Can you work these out from the model? Positions are in its coordinate system, mm. Coordinates: 2 decimals unless noted, no trailing zeros. Order: outer loops, then holes, each group sorted by start corner. A loop starts at its lowest first (then second) coordinate and runs counter-clockwise, first axis right, second up. Notation, with made-up numbers: (71.5, 89) - (127.5, 89) arc R18 cw to (127.5, 95) - close; hole circle Ø11 at (-37.75, 63.5). An arc over 180 degrees is marked (long way). Return JSON: item names as keys, results as strings. Group by question number.
1) If I drill on line 1 along Z through (x, y) = (-0.1, 2); line 2 along Y through (x, z) = (0.15, 4); line 3 along Y through (x, z) = (0.05, 0), over which ranges is the centre line in solid material (lowest first)?
2) Imagine slicing it at A-A (z = 5.75). Write out the boundary of the cut face in (x, y), and give its area (3 significant figures).
3) Imagine slicing it at B-B (y = 8.5). Write out the boundary of the cut face in (x, z), and give its area (3 significant figures).
4) For pin 1 Ø4 at (y, z) = (8.5, 4) entering from -X, with a flat end and sliding along its axis, tell me the tip position at first contact or that it passes through.
Autodesk Inventor part; units mm, degrees
ref_plane "YZ Plane" through (0, 0, 0) normal (1, 0, 0) x (0, 1, 0)
ref_plane "XZ Plane" through (0, 0, 0) normal (0, 1, 0) x (-1, 0, 0)
ref_plane "XY Plane" through (0, 0, 0) normal (0, 0, 1) x (1, 0, 0)
sketch "Sketch1" plane through (0, 0, 0) normal (0, 1, 0) x (-1, 0, 0)
  line L0 (0.2032, -0.381) -> (-0.2032, -0.381)
  line L1 (-0.2032, -0.381) -> (-0.2032, 0.381)
  line L2 (-0.2032, 0.381) -> (0.2032, 0.381)
  line L3 (0.2032, 0.381) -> (0.2032, -0.381)
  line L4 (0.2032, -0.381) -> (-0.2032, 0.381) construction
  line L5 (-0.2032, -0.381) -> (0.2032, 0.381) construction
  point P0 (0, 0)
  dimension "d0" = 0.4064
  dimension "d1" = 0.762
extrude "Extrusion1" add sketch "Sketch1" along normal blind 20.48
chamfer "Chamfer1" distance 0.1 angle 45 8 edges at (0.2032, 20.48, 0) (0, 20.48, -0.381) (0, 20.48, 0.381) (-0.2032, 20.48, 0) (0.2032, 0, 0) (0, 0, -0.381) (0, 0, 0.381) (-0.2032, 0, 0)
sketch "Sketch2" plane through (-0.2032, 0.1, 0.381) normal (0, 0, 1) x (1, 0, 0)
  line L0 (-1.0405, 13.38) -> (1.7368, 13.38)
  point P0 (0.2032, -0.1)
  dimension "d7" = 13.48
bend part "Bend Part1" radius 1 angle 90 line through (-1.2437, 13.48, 0.381) along (1, 0, 0) centre toward (0, 0, 1) moving side (0, 1, 0) both sides no
properties part number "PinRight1" material "Gold"
Calculated:
{
 "1": {"line 1": "-0.38 to 0.38", "line 2": "14.48 to 15.24", "line 3": "0 to 14.57"},
 "2": {"outline": "(-0.2, 14.48) - (0.2, 14.48) - (0.2, 15.24) - (-0.2, 15.24) - close", "area": "0.310 mm2"},
 "3": {"outline": "(-0.2, -0.38) - (0.2, -0.38) - (0.2, 0.38) - (-0.2, 0.38) - close", "area": "0.310 mm2"},
 "4": {"pin 1": "through"}
}
